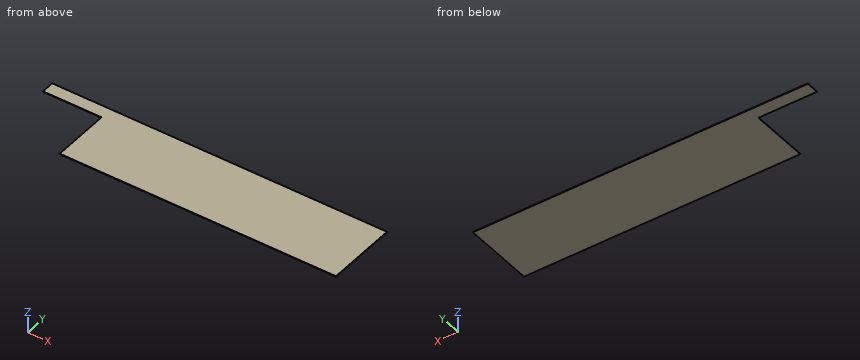
Autodesk Inventor part; units mm, degrees
ref_plane "YZ Plane" through (0, 0, 0) normal (1, 0, 0) x (0, 1, 0)
ref_plane "XZ Plane" through (0, 0, 0) normal (0, 1, 0) x (-1, 0, 0)
ref_plane "XY Plane" through (0, 0, 0) normal (0, 0, 1) x (1, 0, 0)
sketch "Sketch1" plane through (0, 0, 0) normal (0, 0, 1) x (1, 0, 0)
  line L0 (0, 0) -> (2000, 0)
  line L1 (2000, 0) -> (2000, 427)
  line L2 (2000, 427) -> (0, 427)
  line L3 (0, 427) -> (0, 0)
  dimension "d0" = 2000
  dimension "d1" = 427
extrude "Extrusion1" add sketch "Sketch1" along normal blind 3
sketch "Sketch2" plane through (0, 0, 3) normal (0, 0, 1) x (1, 0, 0)
  line L0 (0, 427) -> (0, 0)
  line L1 (0, 0) -> (350, 0)
  line L2 (350, 0) -> (350, 350)
  line L3 (350, 350) -> (0, 350)
  line L4 (0, 350) -> (0, 0)
  point P0 (0, 350)
  dimension "d4" = 350
  dimension "d5" = 350
extrude "Extrusion2" cut sketch "Sketch2" against normal blind 10
properties part number "cover back" material "Nylon 6/6"
Check sheet for the modelled part. Datum: model origin and axes. Units: mm. Give positions to 0.01 mm unless a question says otherwise; leave off trailing zeros. Order: outer loops, then holes, each group sorted by start corner. A loop starts at its lowest first (then second) coordinate and runs counter-clockwise, first axis right, second up. Notation, with made-up numbers: M 54.25,79.5 L 107.25,79.5 A12 cw 107.25,87.5 Z; hole C 4,45 d6. An arc over 180 degrees is marked long. Answer as CSV lines item,"result". Start each with the question number.
Item 1: Gauge pin test, flat end, axial feed: P1, Ø0.9, axis at x = 257.5, z = 1, coming from the -Y side. Record the tip position at first contact, or that the pin passes through.
Item 2: Cross-section at C-C on x = 151. Enter the section's corners in (y, z).
Item 3: Cross-section at B-B on y = 46.5. Enter the section's corners in (x, z).
Item 4: Cross-section at A-A on z = 2.3. Enter the section's corners in (x, y), plus the area to 4 significant figures.
Item 5: Thickness scan on line 1 (Y direction, x = 233, z = 1.05); line 2 (X direction, y = 313, z = 1.1). Record the ranges inside material, lowest first. Write a range as [from, to].
Established:
1,P1,"stops at y = 350"
2,outline,"M 350,0 L 427,0 L 427,3 L 350,3 Z"
3,outline,"M 350,0 L 2000,0 L 2000,3 L 350,3 Z"
4,outline,"M 0,350 L 350,350 L 350,0 L 2000,0 L 2000,427 L 0,427 Z"
4,area,"731,500 mm^2"
5,line 1,"y = [350, 427]"
5,line 2,"x = [350, 2000]"
